Can you work these out from the model? Positions are in its coordinate system, mm. A direction names the side the tool comes from. Round coordinates to 2 decimals unless told otherwise and drop trailing zeros. Write each loop counter-clockwise with the first axis right and the second up, starting at its lowest first coordinate (ties: lowest second). Pieces come first, ordered by that corner, then holes. Notation, with made-up numbers: M 28.5,79 L 32.5,79 A14 cw 32.5,95 Z; hole C 5,22 d7. An arc over 180 degrees is marked long. Answer in a Markdown table with one row per item. Add a question column.
(1) Suppose I cut it at A-A, the plane z = -10.5. Write out the boundary of the cut face in (x, y).
(2) I'm going to push flat-ended pins straight in: pin 1 (8 mm diameter, centred on y = -10.5, z = 3.5, fed in from +X); pin 2 (1.7 mm diameter, centred on x = 9.5, z = -10.5, fed in from -Y). Where does each tip first touch, or does it pass through?
(3) For faces 5 (the face through (-19.5, 0, 0)), 6 (the face through (-9, -6, -11)), 7 (the face through (0, -14, 0)), 8 (the face through (34.444, -3.905, 0.867)), 9 (the face through (30.5, -1, -1)), which set-ups out of +Z, -Z, +X, -X, +Y, -Y let a thin tool reach every point of the face, with its end or its side?
(4) Suppose I cut it at C-C, the plane z = 2.75. Write out the boundary of the cut face in (x, y).
(5) If we mould it in two halves opening along X, with no side actions, what happens to faces 1 (the face through (-9, -6, 10)), 2 (the face through (-10.35, -10.06, 9.39)), 3 (the face through (38.5, 0, 0)), 4 (the face through (0, 14, 0))? For each: released by +X, released by -X, zero draft, split by the parting line, or undercut.
(6) If I drill on probe 1 along X at (y, z) = (-11, 10.5); probe 2 along X at (y, z) = (-8.5, 10); probe 3 along X at (y, z) = (7, -9), over which ranges is the centre line in solid material (lowest first)?
(7) Suppose I cut it at D-D, the plane y = -5. Write out the boundary of the cut face in (x, z), then the cut area to 3 significant figures.
(8) Suppose I cut it at B-B, the plane y = 0. Write out the boundary of the cut face in (x, z), then the cut area to 3 significant figures.
from build123d import *

# Parameters (mm, degrees)
SKETCH2_W           = 39
SKETCH2_H           = 24
BOSS_EXTRUDE1_DEPTH = 14
SKETCH3_R           = 1
BOSS_EXTRUDE2_DEPTH = 11
SKETCH4_R           = 4
BOSS_EXTRUDE3_DEPTH = 8
SKETCH5_R           = 1.4
CUT_EXTRUDE3_DEPTH  = 8


with BuildPart() as part:
    # Sketch2 → Boss-Extrude1 (new, symmetric)
    with BuildSketch(Plane(origin=(0, 0, 0), x_dir=(1, 0, 0), z_dir=(0, 1, 0))):
        Rectangle(SKETCH2_W, SKETCH2_H)
    extrude(amount=BOSS_EXTRUDE1_DEPTH, both=True)

    # Sketch3 → Boss-Extrude2 (add)
    with BuildSketch(Plane(origin=(19.5, 0, 0), x_dir=(0, 0, -1), z_dir=(1, 0, 0))):
        with Locations(Location((0, 0, 0), (0, 0, 180))):
            Circle(SKETCH3_R)
    extrude(amount=BOSS_EXTRUDE2_DEPTH)

    # Sketch4 → Boss-Extrude3 (add)
    with BuildSketch(Plane(origin=(30.5, 0, 0), x_dir=(0, 0, -1), z_dir=(1, 0, 0))):
        Circle(SKETCH4_R)
    extrude(amount=BOSS_EXTRUDE3_DEPTH)

    # Sketch5 → Cut-Extrude3 (cut)
    with BuildSketch(Plane(origin=(0, -14, 0), x_dir=(1, 0, 0), z_dir=(0, 1, 0))):
        with Locations(Location((-9.5, 10.5, 0), (0, 0, 270))):
            Circle(SKETCH5_R)
        with Locations(Location((-9.5, -10.5, 0), (0, 0, 270))):
            Circle(SKETCH5_R)
        with Locations(Location((9.5, 10.5, 0), (0, 0, 270))):
            Circle(SKETCH5_R)
        with Locations(Location((9.5, -10.5, 0), (0, 0, 270))):
            Circle(SKETCH5_R)
    extrude(amount=CUT_EXTRUDE3_DEPTH, mode=Mode.SUBTRACT)


solid = part.part
Calculated:
| question | item | result |
|---|---|---|
| 1 | outline | M -19.5,-14 L -10.9,-14 L -10.9,-6 L -8.1,-6 L -8.1,-14 L 8.1,-14 L 8.1,-6 L 10.9,-6 L 10.9,-14 L 19.5,-14 L 19.5,14 L -19.5,14 Z |
| 2 | pin 1 | x = 19.5 |
| 2 | pin 2 | y = -6 |
| 3 | face 5 | +Z, -Z, -X, +Y, -Y |
| 3 | face 6 | -Y |
| 3 | face 7 | +Z, -Z, +X, -X, -Y |
| 3 | face 8 | +X |
| 3 | face 9 | none |
| 4 | outline | M -19.5,-14 L 19.5,-14 L 19.5,14 L -19.5,14 Z; M 30.5,-2.9 L 38.5,-2.9 L 38.5,2.9 L 30.5,2.9 Z |
| 5 | face 1 | undercut |
| 5 | face 2 | undercut |
| 5 | face 3 | released by +X |
| 5 | face 4 | zero draft |
| 6 | probe 1 | -19.5 to -10.9, -8.1 to 8.1, 10.9 to 19.5 |
| 6 | probe 2 | -19.5 to -10.81, -8.19 to 8.19, 10.81 to 19.5 |
| 6 | probe 3 | -19.5 to 19.5 |
| 7 | outline | M -19.5,-12 L 19.5,-12 L 19.5,12 L -19.5,12 Z |
| 7 | area | 936 mm² |
| 8 | outline | M -19.5,-12 L 19.5,-12 L 19.5,-1 L 30.5,-1 L 30.5,-4 L 38.5,-4 L 38.5,4 L 30.5,4 L 30.5,1 L 19.5,1 L 19.5,12 L -19.5,12 Z |
| 8 | area | 1,020 mm² |
